For this review, take the finished solid that the model builds, in its own axes (mm). Face numbers are marked on the shaded views. A direction names the side the tool comes from. Coordinates: 2 decimals unless noted, no trailing zeros. Write each loop counter-clockwise with the first axis right and the second up, starting at its lowest first coordinate (ties: lowest second). Pieces come first, ordered by that corner, then holes. Notation, with made-up numbers: (-11, 47) -> (17, 47) arc R17 cw to (17, 70) -> close; hole circle Ø8 at (35, 0). An arc over 180 degrees is marked (long way). One line per item, written item: value. Start each with the question number.
1) Add section B-B (y = 8). State the section outline as (x, z) points.
2) Mouldability with a two-part tool opening along Z and no side actions: class the marked faces 1, 2 and 3 as released by +Z, released by -Z, zero draft, split by the parting line, or undercut.
3) Machinability: for the marked faces 4, 5 and 6, which of the approach directions +Z, -Z, +X, -X, +Y, -Y give a long, thin tool a straight path to every point of the face, cutting with its end or side? Answer none if there is none.
4) For pin 1 Ø5.5 at (x, z) = (0, 0) entering from +Y; pin 2 Ø1.5 at (x, y) = (5.5, 29) entering from -Z; pin 3 Ø2 at (y, z) = (32, 4.5) entering from -X, all flat-tipped, find the tip position at first contact; note any pin that passes through.
5) Add section A-A (y = 40). State the section outline as (x, z) points.
6) For probe 1 along Z at (x, y) = (0, -0.8); probe 2 along Z at (x, y) = (0, 40), list the stretches that pass through material, from the lowest coordinate up. Write a range as from..to.
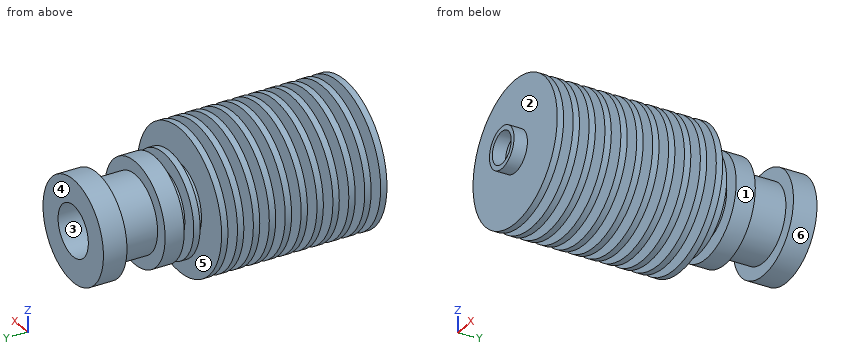
from build123d import *

# Parameters (mm, degrees)
SKETCH2_W           = 8.15
SKETCH2_H           = 1
LPATTERN1_COUNT     = 11
LPATTERN1_PITCH     = 2.5
SKETCH4_R           = 3.25
BOSS_EXTRUDE1_DEPTH = 2.1
SKETCH5_R           = 2.5
CUT_EXTRUDE1_DEPTH  = 2.1


with BuildPart() as part:
    # Sketch1 → Revolve1 (revolve)
    with BuildSketch(Plane.XY):
        Polygon((3, 0), (3, 15.1), (2.1, 15.730186784), (2.1, 34.869605677), (4, 36.2), (4, 42.7), (8, 42.7), (8, 39), (6, 39), (6, 33), (8, 33), (8, 30), (5.5, 30), (8, 0), align=None)
    revolve(axis=Axis((0, 0, 0), (0, 1, 0)))

    # Sketch2 → Revolve2 (revolve)
    with BuildSketch(Plane.XY):
        with Locations((7.075, 0.5)):
            Rectangle(SKETCH2_W, SKETCH2_H)
    revolve2 = revolve(axis=Axis((0, 0, 0), (0, 1, 0)))

    # LPattern1: Revolve2 ×11
    with Locations(*[(0, i * LPATTERN1_PITCH, 0) for i in range(1, LPATTERN1_COUNT)]):
        add(revolve2)

    # Sketch3 → Revolve3 (revolve)
    with BuildSketch(Plane.XY):
        Polygon((5.625, 28.5), (8, 28.5), (8, 27.5), (5.708333333, 27.5), align=None)
    revolve(axis=Axis((0, 0, 0), (0, -1, 0)))

    # Sketch4 → Boss-Extrude1 (add)
    with BuildSketch(Plane.XZ):
        Circle(SKETCH4_R)
    extrude(amount=BOSS_EXTRUDE1_DEPTH)

    # Sketch5 → Cut-Extrude1 (cut)
    with BuildSketch(Plane.XZ.offset(2.1)):
        Circle(SKETCH5_R)
    extrude(amount=-CUT_EXTRUDE1_DEPTH, mode=Mode.SUBTRACT)


solid = part.part
Numbers:
1. outline: circle Ø22.3 at (0, 0); hole circle Ø6 at (0, 0)
2. face 1: split by the parting line
2. face 2: zero draft
2. face 3: undercut
3. face 4: +Z, -Z, +X, -X, +Y
3. face 5: none
3. face 6: +Y
4. pin 1: y = 35.32
4. pin 2: z = -6.29
4. pin 3: x = -7.19
5. outline: circle Ø16 at (0, 0); hole circle Ø8 at (0, 0)
6. probe 1: -3.25..-2.5, 2.5..3.25
6. probe 2: -8..-4, 4..8
